Verification items for the finished model (mm, model axes). A direction names the side the tool comes from. Give positions to 0.01 mm unless a question says otherwise; leave off trailing zeros. Write each loop counter-clockwise with the first axis right and the second up, starting at its lowest first coordinate (ties: lowest second). Pieces come first, ordered by that corner, then holes.
from build123d import *

# Parameters (mm, degrees)
BOSS_EXTRUDE1_DEPTH = 4.25
CUT_EXTRUDE1_DEPTH  = 2.5
SKETCH3_W           = 31.35
SKETCH3_H           = 3
BOSS_EXTRUDE2_DEPTH = 20
FILLET1_R           = 1
SWEEP1_START        = -65.5
SWEEP1_DEPTH        = 55
SKETCH6_W           = 2
SKETCH6_H           = 50
BOSS_EXTRUDE3_DEPTH = 2.5
RIB1_REACH          = 151.987
SKETCH7_WALL_W      = 311.873243788
SKETCH7_WALL_H      = 2
BOSS_EXTRUDE4_DEPTH = 16
FILLET2_R           = 2


# Read off the part's stored shape, not the designer's step: Sweep1
with BuildPart() as part:
    # Sketch1 → Boss-Extrude1 (new body)
    with BuildSketch(Plane(origin=(0, 0, 0), x_dir=(1, 0, 0), z_dir=(0, 1, 0))):
        with BuildLine():
            Line((0, 0), (147, 0))
            ThreePointArc((147, 0), (149.121320344, 0.878679656), (150, 3))
            Line((150, 3), (150, 73))
            ThreePointArc((150, 73), (149.121320344, 75.121320344), (147, 76))
            Line((147, 76), (0, 76))
            Line((0, 76), (0, 0))
        make_face()
    extrude(amount=BOSS_EXTRUDE1_DEPTH)

    # Sketch2 → Cut-Extrude1 (cut)
    with BuildSketch(Plane(origin=(0, 4.25, 0), x_dir=(1, 0, 0), z_dir=(0, 1, 0))):
        with BuildLine():
            Line((0, 74.875), (145.875, 74.875))
            ThreePointArc((145.875, 74.875), (147.996320344, 73.996320344), (148.875, 71.875))
            Line((148.875, 71.875), (148.875, 4.125))
            ThreePointArc((148.875, 4.125), (147.996320344, 2.003679656), (145.875, 1.125))
            Line((145.875, 1.125), (0, 1.125))
            Line((0, 1.125), (0, 74.875))
        make_face()
    extrude(amount=-CUT_EXTRUDE1_DEPTH, mode=Mode.SUBTRACT)

    # Sketch3 → Boss-Extrude2 (add)
    with BuildSketch(Plane(origin=(0, 0, 0), x_dir=(1, 0, 0), z_dir=(0, 1, 0))):
        with Locations((22.25, 74.5)):
            Rectangle(SKETCH3_W, SKETCH3_H)
    extrude(amount=BOSS_EXTRUDE2_DEPTH)

    # Fillet1
    fillet1_edges = [part.edges().sort_by_distance(p)[0] for p in [
        (73.5, 0, 0),
        (149.121320344, 0, -0.878679656),
        (150, 0, -38),
        (149.121320344, 0, -75.121320344),
        (73.5, 0, -76),
    ]]
    fillet(fillet1_edges, radius=FILLET1_R)

    # Sweep1 outline → Sweep1 (add)
    with BuildSketch(Plane.XY.offset(SWEEP1_START)):
        with BuildLine():
            Line((0, 3.75), (-2, 3.75))
            Line((-2, 3.75), (-2, 1.75))
            Line((-2, 1.75), (2, 1.75))
            ThreePointArc((2, 1.75), (1.414213562, 3.164213562), (0, 3.75))
        make_face()
    extrude(amount=SWEEP1_DEPTH)

    # Sketch6 → Boss-Extrude3 (add)
    with BuildSketch(Plane(origin=(0, 1.75, 0), x_dir=(1, 0, 0), z_dir=(0, 1, 0))):
        with Locations((146.575, 38)):
            Rectangle(SKETCH6_W, SKETCH6_H)
    extrude(amount=BOSS_EXTRUDE3_DEPTH)

    # Sketch7 wall → Rib1 (add, up to next)
    with BuildSketch(Plane(origin=(22.25, 5.25, -69.5), x_dir=(0, -0.707106781187, 0.707106781187), z_dir=(0, 0.707106781187, 0.707106781187)), mode=Mode.PRIVATE) as rib1_sk1:
        Rectangle(SKETCH7_WALL_W, SKETCH7_WALL_H)
    rib1_tool1 = extrude(rib1_sk1.sketch, amount=-RIB1_REACH, mode=Mode.PRIVATE) - part.part
    add(rib1_tool1.solids().sort_by_distance((22.25, 5.25, -69.5))[0])

    # Sketch8 → Boss-Extrude4 (add)
    with BuildSketch(Plane(origin=(0, 1.75, 0), x_dir=(1, 0, 0), z_dir=(0, 1, 0))):
        with BuildLine():
            Line((127.05753899, 42), (127.05753899, 34))
            ThreePointArc((127.05753899, 34), (124.55753899, 31.5), (122.05753899, 34))
            Line((122.05753899, 34), (122.05753899, 42))
            ThreePointArc((122.05753899, 42), (124.55753899, 44.5), (127.05753899, 42))
        make_face()
    extrude(amount=BOSS_EXTRUDE4_DEPTH)

    # Fillet2
    fillet2_edges = [part.edges().sort_by_distance(p)[0] for p in [
        (124.55753899, 1.75, -44.5),
        (122.05753899, 1.75, -38),
        (124.55753899, 1.75, -31.5),
        (127.05753899, 1.75, -38),
    ]]
    fillet(fillet2_edges, radius=FILLET2_R)


solid = part.part
Item 1: Depth check by flat-ended pin: pin 1 (2 mm diameter, centred on x = 63.5, z = -62, fed in from +Y); pin 2 (9 mm diameter, centred on y = 11, z = -37.5, fed in from +X); pin 3 (2 mm diameter, centred on x = -1, z = -44, fed in from +Y). Enter the tip coordinate at first touch or a pass-through.
Answer key:
pin 1: stops at y = 1.75
pin 2: stops at x = 127.06
pin 3: stops at y = 3.75
Item 2: Release check for a two-part mould opening along Z. For faces 1 (the face through (22, 20, -75)), 2 (the face through (75, 1.75, -39)), 3 (the face through (72, 3, 0)) record: released by +Z, released by -Z, zero draft, split by the parting line, or undercut.
Answer key:
face 1: zero draft
face 2: undercut
face 3: released by +Z
Item 3: Sectioned sample at B-B on x = 73. Record the cut outline in (y, z) (3 decimals).
Answer key:
outline: (0, -75) arc R1 ccw to (1, -76) - (4.25, -76) - (4.25, -74.875) - (1.75, -74.875) - (1.75, -1.125) - (4.25, -1.125) - (4.25, 0) - (1, 0) arc R1 ccw to (0, -1) - close
Item 4: Scan lines: line 1 along X through (y, z) = (3.75, -71) (3 decimals); line 2 along Y through (x, z) = (15.5, -66); line 3 along Z through (x, y) = (16, 7.5). Record each from-to range of solid material in increasing order.
Answer key:
line 1: x = 21.25 to 23.25, 148.875 to 150
line 2: y = 0 to 1.75
line 3: z = -76 to -73
Item 5: Sectioned sample at A-A on z = -25. Record the cut outline in (x, y) (3 decimals).
Answer key:
outline: (-2, 1.75) - (0, 1.75) - (0, 0) - (149, 0) arc R1 ccw to (150, 1) - (150, 4.25) - (148.875, 4.25) - (148.875, 1.75) - (147.575, 1.75) - (147.575, 4.25) - (145.575, 4.25) - (145.575, 1.75) - (2, 1.75) arc R2 ccw to (0, 3.75) - (-2, 3.75) - close
Item 6: Set-up check for faces 4 (the face through (147.97, 3.02, -74.02)), 5 (the face through (149.1, 2.6, -0.86)), 6 (the face through (21.25, 4, -71)): record each of +Z, -Z, +X, -X, +Y, -Y from which the full face is reachable in a straight line by a thin tool's end or side.
Answer key:
face 4: +Y
face 5: +Z, +X, +Y, -Y
face 6: -X, +Y
Item 7: Sectioned sample at C-C on z = -37. Record the cut outline in (x, y) (3 decimals).
Answer key:
outline: (-2, 1.75) - (0, 1.75) - (0, 0) - (149, 0) arc R1 ccw to (150, 1) - (150, 4.25) - (148.875, 4.25) - (148.875, 1.75) - (147.575, 1.75) - (147.575, 4.25) - (145.575, 4.25) - (145.575, 1.75) - (129.058, 1.75) arc R2 cw to (127.058, 3.75) - (127.058, 17.75) - (122.058, 17.75) - (122.058, 3.75) arc R2 cw to (120.058, 1.75) - (2, 1.75) arc R2 ccw to (0, 3.75) - (-2, 3.75) - close
